Source: CAD feature listing. Evaluate the final solid. Frame: model axes, mm. Face numbers are marked on the shaded views. A direction names the side the tool comes from. Give positions to 0.01 mm unless a question says otherwise; leave off trailing zeros. Loops run counter-clockwise (first coordinate to the right, second up) from the corner with the lowest first, then second, coordinate; pieces in that order, holes last. Notation, with made-up numbers: M 25.25,19 L 75.25,19 A27 cw 75.25,39 Z; hole C 19.25,3 d2. An arc over 180 degrees is marked long. Answer in a Markdown table with one row per item.
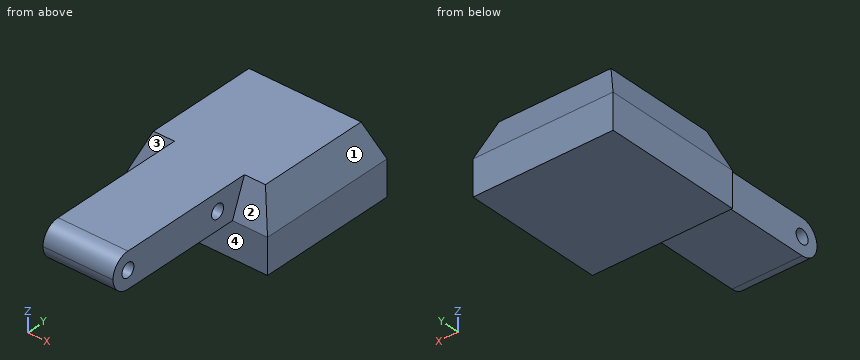
```python
from build123d import *

# Parameters (mm, degrees)
CROQUIS1_W              = 20
CROQUIS1_H              = 40
SALIENTE_EXTRUIR1_DEPTH = 10
CROQUIS2_R              = 2
CORTAR_EXTRUIR1_DEPTH   = 31
CROQUIS3_W              = 40
CROQUIS3_H              = 10
SALIENTE_EXTRUIR2_DEPTH = 10
CROQUIS4_W              = 40
CROQUIS4_H              = 40
SALIENTE_EXTRUIR3_DEPTH = 20
CORTAR_EXTRUIR3_DEPTH   = 10
CORTAR_EXTRUIR4_DEPTH   = 10
CORTAR_EXTRUIR5_DEPTH   = 41
CORTAR_EXTRUIR6_DEPTH   = 40
CORTAR_EXTRUIR7_DEPTH   = 31


with BuildPart() as part:
    # Croquis1 → Saliente-Extruir1 (new body)
    with BuildSketch(Plane.XY):
        Rectangle(CROQUIS1_W, CROQUIS1_H)
        Polygon((0, 20), (10, 20), (20, 20), (20, 50), (0, 50), align=None)
        Polygon((-20, 20), (-10, 20), (0, 20), (0, 50), (-20, 50), align=None)
    extrude(amount=SALIENTE_EXTRUIR1_DEPTH)

    # Croquis2 → Cortar-Extruir1 (cut, through all)
    with BuildSketch(Plane(origin=(10, 0, 0), x_dir=(0, 0, -1), z_dir=(1, 0, 0))):
        with Locations((-5, -15)):
            Circle(CROQUIS2_R)
        with Locations((-5, 15)):
            Circle(CROQUIS2_R)
    extrude(amount=-CORTAR_EXTRUIR1_DEPTH, mode=Mode.SUBTRACT)

    # Croquis3 → Saliente-Extruir2 (add)
    with BuildSketch(Plane(origin=(0, 50, 0), x_dir=(1, 0, 0), z_dir=(0, 1, 0))):
        with Locations((0, -5)):
            Rectangle(CROQUIS3_W, CROQUIS3_H)
    extrude(amount=SALIENTE_EXTRUIR2_DEPTH)

    # Croquis4 → Saliente-Extruir3 (add)
    with BuildSketch(Plane.XY.offset(10)):
        with Locations((0, 40)):
            Rectangle(CROQUIS4_W, CROQUIS4_H)
    extrude(amount=-SALIENTE_EXTRUIR3_DEPTH)

    # Croquis6 → Cortar-Extruir3 (cut)
    with BuildSketch(Plane(origin=(20, 0, 0), x_dir=(0, 0, -1), z_dir=(1, 0, 0))):
        Polygon((-10, 20), (0, 20), (-10, 24), align=None)
    extrude(amount=-CORTAR_EXTRUIR3_DEPTH, mode=Mode.SUBTRACT)

    # Croquis7 → Cortar-Extruir4 (cut)
    with BuildSketch(Plane.ZY.offset(20)):
        Polygon((0, 20), (10, 24), (10, 20), align=None)
    extrude(amount=-CORTAR_EXTRUIR4_DEPTH, mode=Mode.SUBTRACT)

    # Croquis8 → Cortar-Extruir5 (cut, through all)
    with BuildSketch(Plane(origin=(20, 0, 0), x_dir=(0, 0, -1), z_dir=(1, 0, 0))):
        Polygon((-10, 56), (0, 60), (-10, 60), align=None)
    extrude(amount=-CORTAR_EXTRUIR5_DEPTH, mode=Mode.SUBTRACT)

    # Croquis9 → Cortar-Extruir6 (cut)
    with BuildSketch(Plane(origin=(0, 60, 0), x_dir=(1, 0, 0), z_dir=(0, 1, 0))):
        Polygon((-20, 0), (-20, -10), (-16, -10), align=None)
        Polygon((20, 0), (20, -10), (16, -10), align=None)
    extrude(amount=-CORTAR_EXTRUIR6_DEPTH, mode=Mode.SUBTRACT)

    # Croquis10 → Cortar-Extruir7 (cut, through all)
    with BuildSketch(Plane(origin=(10, 0, 0), x_dir=(0, 0, -1), z_dir=(1, 0, 0))):
        with BuildLine():
            ThreePointArc((0, -15), (-1.464466094, -18.535533906), (-5, -20))
            Line((-5, -20), (0, -20))
            Line((0, -20), (0, -15))
        make_face()
        with BuildLine():
            ThreePointArc((-5, -20), (-8.535533906, -18.535533906), (-10, -15))
            Line((-10, -15), (-10, -20))
            Line((-10, -20), (-5, -20))
        make_face()
    extrude(amount=-CORTAR_EXTRUIR7_DEPTH, mode=Mode.SUBTRACT)


solid = part.part
```
Q1. Contact query for flat-ended pins moving along their axis: pin 1 Ø5 at (x, y) = (14.5, 0.5) entering from -Z; pin 2 Ø6.5 at (y, z) = (15, 5) entering from -X; pin 3 Ø4 at (x, z) = (4.5, -4) entering from -Y; pin 4 Ø4 at (x, z) = (6.5, 2.5) entering from +Y. Output: stop coordinate, or through.
Values follow:
| item | result |
|---|---|
| pin 1 | through |
| pin 2 | x = -10 |
| pin 3 | y = 20 |
| pin 4 | y = 59.8 |
Q2. Reachability of the marked faces 1, 2, 3 and 4 from +Z, -Z, +X, -X, +Y, -Y: full face, straight path, thin tool, end or side. Return the list, or none.
Values follow:
| item | result |
|---|---|
| face 1 | +Z, +X, +Y, -Y |
| face 2 | +Z, +X, -Y |
| face 3 | +Z, -X, -Y |
| face 4 | -Z, +X, -X, -Y |
Q3. Section query C-C (y = 55). Output: boundary loops of the cut face in (x, z).
Values follow:
| item | result |
|---|---|
| outline | M -20,-10 L 20,-10 L 20,0 L 16,10 L -16,10 L -20,0 Z |
Q4. Section query B-B (y = 15). Output: boundary loops of the cut face in (x, z), plus the area to 3 significant figures.
Values follow:
| item | result |
|---|---|
| outline | M -10,0 L 10,0 L 10,3 L -10,3 Z; M -10,7 L 10,7 L 10,10 L -10,10 Z |
| area | 120 mm^2 |
Q5. Ray query, probe 1 along Y at (x, z) = (-2.5, 5); probe 2 along X at (y, z) = (-2, 8); probe 3 along Y at (x, z) = (17.5, -8). Return the intervals inside material, ascending. Write a range as from..to.
Values follow:
| item | result |
|---|---|
| probe 1 | -20..-17, -13..13, 17..58 |
| probe 2 | -10..10 |
| probe 3 | 20..60 |
Q6. Section query D-D (z = -4.5). Output: boundary loops of the cut face in (x, y).
Values follow:
| item | result |
|---|---|
| outline | M -20,20 L 20,20 L 20,60 L -20,60 Z |
Q7. Section query A-A (x = -7.5). Output: boundary loops of the cut face in (y, z), plus the area to 3 significant figures.
Values follow:
| item | result |
|---|---|
| outline | M -15,0 L 20,0 L 20,-10 L 60,-10 L 60,0 L 56,10 L -15,10 A5 ccw Z; hole C -15,5 d4; hole C 15,5 d4 |
| area | 1,140 mm^2 |
